from build123d import *

# Parameters (mm, degrees)
SKETCH1_W           = 120
SKETCH1_H           = 100
BOSS_EXTRUDE1_DEPTH = 3
SKETCH2_W           = 10
SKETCH2_H           = 3
SKETCH2_W_2         = 20
BOSS_EXTRUDE3_DEPTH = 3
SKETCH3_W           = 10
SKETCH3_H           = 3
SKETCH3_W_2         = 20
BOSS_EXTRUDE4_DEPTH = 3
SKETCH5_W           = 80
SKETCH5_H           = 106
CUT_EXTRUDE1_DEPTH  = 3
SKETCH6_R           = 1.5
CUT_EXTRUDE2_DEPTH  = 10
SKETCH7_W           = 19.608717555
SKETCH7_H           = 29.132951796
CUT_EXTRUDE3_DEPTH  = 10


with BuildPart() as part:
    # Sketch1 → Boss-Extrude1 (new body)
    with BuildSketch(Plane(origin=(0, 0, 0), x_dir=(1, 0, 0), z_dir=(0, 1, 0))):
        with Locations((60, 50)):
            Rectangle(SKETCH1_W, SKETCH1_H)
    extrude(amount=BOSS_EXTRUDE1_DEPTH)

    # Sketch2 → Boss-Extrude3 (add)
    with BuildSketch(Plane(origin=(0, 3, 0), x_dir=(1, 0, 0), z_dir=(0, 1, 0))):
        with Locations((5, -1.5)):
            Rectangle(SKETCH2_W, SKETCH2_H)
        with Locations((40, -1.5)):
            Rectangle(SKETCH2_W_2, SKETCH2_H)
        with Locations((80, -1.5)):
            Rectangle(SKETCH2_W_2, SKETCH2_H)
        with Locations((115, -1.5)):
            Rectangle(SKETCH2_W, SKETCH2_H)
    extrude(amount=-BOSS_EXTRUDE3_DEPTH)

    # Sketch3 → Boss-Extrude4 (add)
    with BuildSketch(Plane.XZ):
        with Locations((5, -101.5)):
            Rectangle(SKETCH3_W, SKETCH3_H)
        with Locations((40, -101.5)):
            Rectangle(SKETCH3_W_2, SKETCH3_H)
        with Locations((80, -101.5)):
            Rectangle(SKETCH3_W_2, SKETCH3_H)
        with Locations((115, -101.5)):
            Rectangle(SKETCH3_W, SKETCH3_H)
    extrude(amount=-BOSS_EXTRUDE4_DEPTH)

    # Sketch5 → Cut-Extrude1 (cut)
    with BuildSketch(Plane.XZ):
        with Locations((80, -50)):
            Rectangle(SKETCH5_W, SKETCH5_H)
    extrude(amount=-CUT_EXTRUDE1_DEPTH, mode=Mode.SUBTRACT)

    # Sketch6 → Cut-Extrude2 (cut)
    with BuildSketch(Plane.XZ):
        with Locations((30, -74.938410105)):
            Circle(SKETCH6_R)
        with BuildLine():
            Line((31.476820396, -26.938410105), (31.476820396, -22.938410105))
            ThreePointArc((31.476820396, -22.938410105), (29.976820396, -21.438410105), (28.476820396, -22.938410105))
            Line((28.476820396, -22.938410105), (28.476820396, -26.938410105))
            ThreePointArc((28.476820396, -26.938410105), (29.976820396, -28.438410105), (31.476820396, -26.938410105))
        make_face()
    extrude(amount=-CUT_EXTRUDE2_DEPTH, mode=Mode.SUBTRACT)

    # Sketch7 → Cut-Extrude3 (cut)
    with BuildSketch(Plane.XZ):
        with Locations((24.804358778, -50)):
            Rectangle(SKETCH7_W, SKETCH7_H)
    extrude(amount=-CUT_EXTRUDE3_DEPTH, mode=Mode.SUBTRACT)


solid = part.part
For this review, take the finished solid that the model builds, in its own axes (mm). A direction names the side the tool comes from. Round coordinates to 2 decimals unless told otherwise and drop trailing zeros. Loops run counter-clockwise (first coordinate to the right, second up) from the corner with the lowest first, then second, coordinate; pieces in that order, holes last. Notation, with made-up numbers: (55, -13.5) - (83, -13.5) arc R34 cw to (83, 24.5) - close; hole circle Ø8 at (58, 88). An arc over 180 degrees is marked (long way). Use one line per item in the form item = value.
1) We need section A-A on z = -47. Write out the cut boundary in (x, y), then the cut area to 3 significant figures.
Solutions:
outline = (0, 0) - (15, 0) - (15, 3) - (0, 3) - close; (34.61, 0) - (40, 0) - (40, 3) - (34.61, 3) - close
area = 61.2 mm2
2) Tool access review of faces 1 (the face through (20, 1, -100)), 2 (the face through (30, 2, 2)), 3 (the face through (40, 1, -51)), 4 (the face through (34.609, 1, -50)): name each direction out of +Z, -Z, +X, -X, +Y, -Y from which nothing blocks a thin tool from reaching the whole face with its end or side.
Solutions:
face_1 = -Z, +Y, -Y
face_2 = +Z, +Y, -Y
face_3 = +Z, -Z, +X, +Y, -Y
face_4 = +Y, -Y
3) Clearance check with flat-ended pins moving along their axes: P1, Ø1.5, axis at y = 1.5, z = -25.5, coming from the -X side; P2, Ø1.5, axis at x = 18.5, y = 2, coming from the +Z side; P3, Ø1, axis at x = 12, y = 2.5, coming from the -Z side. State where each tip first meets the part, or that it passes through.
Solutions:
P1 = 0
P2 = 0
P3 = -100
4) We need section C-C on y = 1. Write out the cut boundary in (x, z).
Solutions:
outline = (0, -103) - (10, -103) - (10, -100) - (30, -100) - (30, -103) - (40, -103) - (40, 3) - (30, 3) - (30, 0) - (10, 0) - (10, 3) - (0, 3) - close; hole (15, -64.57) - (34.61, -64.57) - (34.61, -35.43) - (15, -35.43) - close; hole (28.48, -26.94) arc R1.5 ccw to (31.48, -26.94) - (31.48, -22.94) arc R1.5 ccw to (28.48, -22.94) - close; hole circle Ø3 at (30, -74.94)
5) Mouldability with a two-part tool opening along X and no side actions: class faces 5 (the face through (0, 1, -51)), 6 (the face through (10, 1, -102)), 7 (the face through (11, 3, -49)) as pulls with the +X half, pulls with the -X half, needs draft (parallel to the pull), parting line crosses it, or undercut.
Solutions:
face_5 = pulls with the -X half
face_6 = undercut
face_7 = needs draft
6) We need section B-B on x = 25.5. Write out the cut boundary in (y, z), then the cut area to 3 significant figures.
Solutions:
outline = (0, -100) - (3, -100) - (3, -64.57) - (0, -64.57) - close; (0, -35.43) - (3, -35.43) - (3, 0) - (0, 0) - close
area = 213 mm2
7) Wall thickness on probe 1 along X at (y, z) = (0.2, -56); probe 2 along Z at (x, y) = (30.5, 0.15); probe 3 along X at (y, z) = (0.7, -26): over which ranges is each line inside the solid? List them lowest first.
Solutions:
probe_1 = 0 to 15, 34.61 to 40
probe_2 = -103 to -76.35, -73.52 to -64.57, -35.43 to -28.34, -21.53 to 3
probe_3 = 0 to 28.48, 31.48 to 40
